Part model, mm, in its own coordinate system. A direction names the side the tool comes from. Coordinates: 2 decimals unless noted, no trailing zeros. Order: outer loops, then holes, each group sorted by start corner. A loop starts at its lowest first (then second) coordinate and runs counter-clockwise, first axis right, second up.
from build123d import *

# Parameters (mm, degrees)
SKETCH_1_W                       = 196
SKETCH_1_H                       = 15
SM_BASE_FLANGE_1_DEPTH           = 1
SM_EDGE_FLANGE_1_STRIP_W         = 5.4732
SM_EDGE_FLANGE_1_STRIP_H         = 1
SM_EDGE_FLANGE_1_STRIP_CUT_DEPTH = 15
SM_EDGE_FLANGE_1_DEPTH           = 15
SM_EDGE_FLANGE_2_STRIP_W         = 5.4732
SM_EDGE_FLANGE_2_STRIP_H         = 1
SM_EDGE_FLANGE_2_STRIP_CUT_DEPTH = 15
SM_EDGE_FLANGE_2_DEPTH           = 15


# Sheet-metal steps are written as plain solids
with BuildPart() as part:
    # Sketch 1 → Базовая кромка1 (new body)
    with BuildSketch(Plane(origin=(0, 0, 0), x_dir=(1, 0, 0), z_dir=(0, 1, 0))):
        with Locations((98, 7.5)):
            Rectangle(SKETCH_1_W, SKETCH_1_H)
    extrude(amount=-SM_BASE_FLANGE_1_DEPTH)

    # Ребро-кромка1 strip (across the edge) → Ребро-кромка1 strip cut (cut)
    with BuildSketch(Plane.XY.offset(-15)):
        with Locations((-1, -0.5)):
            Rectangle(SM_EDGE_FLANGE_1_STRIP_W, SM_EDGE_FLANGE_1_STRIP_H)
    extrude(amount=SM_EDGE_FLANGE_1_STRIP_CUT_DEPTH, mode=Mode.SUBTRACT)

    # Ребро-кромка1 section (across the edge) → Ребро-кромка1 (add)
    with BuildSketch(Plane.XY.offset(-15)):
        with BuildLine():
            Line((0, 0.7366), (0, 37.5))
            Line((0, 37.5), (1, 37.5))
            Line((1, 37.5), (1, 0.7366))
            ThreePointArc((1, 0.7366), (1.215745145, 0.215745145), (1.7366, 0))
            Line((1.7366, 0), (1.7366, -1))
            ThreePointArc((1.7366, -1), (0.508638364, -0.491361636), (0, 0.7366))
        make_face()
    extrude(amount=SM_EDGE_FLANGE_1_DEPTH)

    # Ребро-кромка2 strip (across the edge) → Ребро-кромка2 strip cut (cut)
    with BuildSketch(Plane(origin=(196, 0, 0), x_dir=(-1, 0, 0), z_dir=(0, 0, -1))):
        with Locations((-1, -0.5)):
            Rectangle(SM_EDGE_FLANGE_2_STRIP_W, SM_EDGE_FLANGE_2_STRIP_H)
    extrude(amount=SM_EDGE_FLANGE_2_STRIP_CUT_DEPTH, mode=Mode.SUBTRACT)

    # Ребро-кромка2 section (across the edge) → Ребро-кромка2 (add)
    with BuildSketch(Plane(origin=(196, 0, 0), x_dir=(-1, 0, 0), z_dir=(0, 0, -1))):
        with BuildLine():
            Line((0, 0.7366), (0, 37.5))
            Line((0, 37.5), (1, 37.5))
            Line((1, 37.5), (1, 0.7366))
            ThreePointArc((1, 0.7366), (1.215745145, 0.215745145), (1.7366, 0))
            Line((1.7366, 0), (1.7366, -1))
            ThreePointArc((1.7366, -1), (0.508638364, -0.491361636), (0, 0.7366))
        make_face()
    extrude(amount=SM_EDGE_FLANGE_2_DEPTH)


solid = part.part
Q1. Pin check, flat tips, straight feed: pin 1 Ø1.5 at (x, z) = (97.5, -9) entering from +Y; pin 2 Ø6 at (y, z) = (19.5, -9.5) entering from -X. Stop position of each tip, or through.
Results list:
pin 1: stops at y = 0
pin 2: stops at x = 0
Q2. Wall check: line 1 along X through (y, z) = (31, -7.25); line 2 along Y through (x, z) = (36.5, -3). Give the ranges that are in metal, low to high.
Results list:
line 1: x = 0 to 1, 195 to 196
line 2: y = -1 to 0
Q3. Cut at B-B on z = -11. Write the cut outline in (x, y), and give its area (3 significant figures).
Results list:
outline: (0, 0.74) arc R1.74 ccw to (1.74, -1) - (194.26, -1) arc R1.74 ccw to (196, 0.74) - (196, 37.5) - (195, 37.5) - (195, 0.74) arc R0.74 cw to (194.26, 0) - (1.74, 0) arc R0.74 cw to (1, 0.74) - (1, 37.5) - (0, 37.5) - close
area: 270 mm2
Q4. Cut at C-C on x = 119. Write the cut outline in (y, z).
Results list:
outline: (-1, -15) - (0, -15) - (0, 0) - (-1, 0) - close
Q5. Mould opens along X. For faces 1 (the face through (195, 19, -7)), 2 (the face through (97.5, -0.2, 0)), 3 (the face through (0, 19, -8)) say: pulls with the +X half, pulls with the -X half, needs draft (parallel to the pull), parting line crosses it, or undercut.
Results list:
face 1: undercut
face 2: needs draft
face 3: pulls with the -X half
Q6. Which spindle directions (+Z, -Z, +X, -X, +Y, -Y) get a long thin tool onto all of the face, cutting with end or side? Do faces 4 (the face through (1, 19, -8)), 5 (the face through (97.5, -0.2, -15)). Say none if no direction does.
Results list:
face 4: +Z, -Z, +Y
face 5: -Z, +X, -X, +Y, -Y
Q7. Cut at A-A on y = 34. Write the cut outline in (x, z), and give its area (3 significant figures).
Results list:
outline: (0, -15) - (1, -15) - (1, 0) - (0, 0) - close; (195, -15) - (196, -15) - (196, 0) - (195, 0) - close
area: 30.0 mm2
